Here's the drawing with two shaded views (mm, measured from the low corner). I have some questions. A direction names the side the tool comes from. Coordinates: 2 decimals unless noted, no trailing zeros. Write each loop counter-clockwise with the first axis right and the second up, starting at its lowest first coordinate (ties: lowest second). Pieces come first, ordered by that corner, then holes. Notation, with made-up numbers: (16, -17.75) -> (34, -17.75) arc R19 ccw to (34, 6.25) -> close; hole circle Ø4 at (9, -14.75). An arc over 180 degrees is marked (long way). Answer in a Markdown table with one row per item. Add a question column.
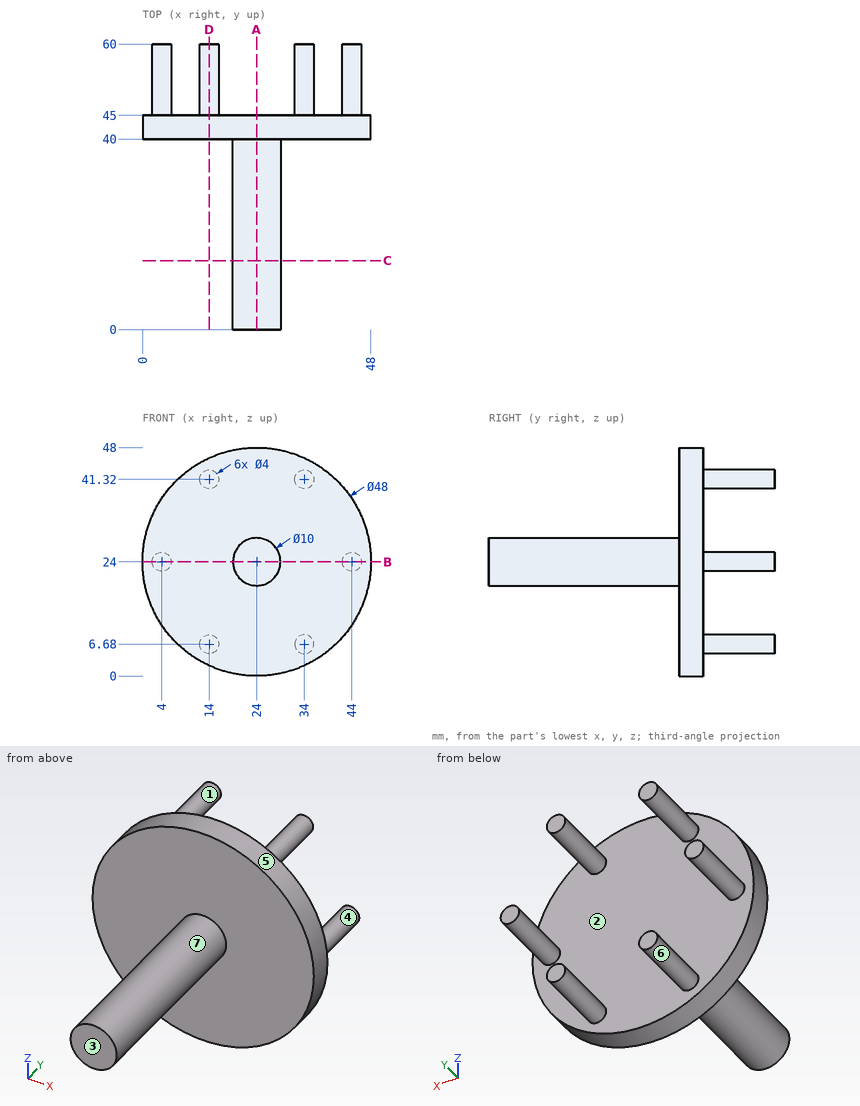
Q1. I need wall thicknesses on line 1 (Y direction, x = 13, z = 28.5); line 2 (X direction, y = 30, z = 25.5); line 3 (Z direction, x = 18, y = 42.5). Which ranges of each line are inside material? Lowest first, please. Write a range as [from, to].
Q2. Imagine slicing it at B-B on z = 24. Please give me the cut outline in (x, y).
Q3. Imagine slicing it at D-D on x = 14. Please give me the cut outline in (y, z).
Q4. I'm going to push flat-ended pins straight in: P1, Ø1, axis at x = 22, y = 32.5, coming from the +Z side; P2, Ø3, axis at x = 35, z = 36.5, coming from the +Y side; P3, Ø8, axis at x = 22.5, y = 32.5, coming from the -Z side. Where does each tip first touch, or does it pass through?
Q5. For the marked faces 5, 6 and 7, which set-ups out of +Z, -Z, +X, -X, +Y, -Y let a thin tool reach every point of the face, with its end or its side?
Q6. If we mould it in two halves opening along Z, with no side actions, what happens to the marked faces 1, 2, 3 and 4? For each: pulls with the +Z half, pulls with the -Z half, needs draft (parallel to the pull), parting line crosses it, or undercut.
Q7. Imagine slicing it at C-C on y = 14.5. Please give me the cut outline in (x, z).
Q8. Imagine slicing it at A-A on x = 24. Please give me the cut outline in (y, z).
Result sheet:
| question | item | result |
|---|---|---|
| 1 | line 1 | y = [40, 45] |
| 1 | line 2 | x = [19.23, 28.77] |
| 1 | line 3 | z = [0.76, 47.24] |
| 2 | outline | (0, 40) -> (19, 40) -> (19, 0) -> (29, 0) -> (29, 40) -> (48, 40) -> (48, 45) -> (46, 45) -> (46, 60) -> (42, 60) -> (42, 45) -> (6, 45) -> (6, 60) -> (2, 60) -> (2, 45) -> (0, 45) -> close |
| 3 | outline | (40, 2.18) -> (45, 2.18) -> (45, 4.68) -> (60, 4.68) -> (60, 8.68) -> (45, 8.68) -> (45, 39.32) -> (60, 39.32) -> (60, 43.32) -> (45, 43.32) -> (45, 45.82) -> (40, 45.82) -> close |
| 4 | P1 | stops at z = 28.77 |
| 4 | P2 | stops at y = 45 |
| 4 | P3 | stops at z = 19 |
| 5 | face 5 | +Y, -Y |
| 5 | face 6 | +Y |
| 5 | face 7 | -Y |
| 6 | face 1 | undercut |
| 6 | face 2 | undercut |
| 6 | face 3 | needs draft |
| 6 | face 4 | parting line crosses it |
| 7 | outline | circle Ø10 at (24, 24) |
| 8 | outline | (0, 19) -> (40, 19) -> (40, 0) -> (45, 0) -> (45, 48) -> (40, 48) -> (40, 29) -> (0, 29) -> close |
